Verification items for the finished model (mm, model axes). A direction names the side the tool comes from. Give positions to 0.01 mm unless a question says otherwise; leave off trailing zeros. Write each loop counter-clockwise with the first axis right and the second up, starting at its lowest first coordinate (ties: lowest second). Pieces come first, ordered by that corner, then holes. Notation, with made-up numbers: M 87,11.5 L 128,11.5 A12 cw 128,24.5 Z; hole C 16.5,52.25 d9. An arc over 180 degrees is marked long. Answer as a JSON object with one key per item and string values.
```python
from build123d import *

# Parameters (mm, degrees)
F0_W          = 76.2
F0_H          = 50.8
F1_DEPTH      = 50.8
F2_R          = 5.08
F3_R          = 6.35
F4_DEPTH      = 25.4
F4_DEPTH_BACK = 25.4
F5_SIZE       = 5.08


with BuildPart() as f1:
    # F0 (on Front) → F1 (new body)
    with BuildSketch(Plane.XZ):
        with Locations((38.1, 25.4)):
            Rectangle(F0_W, F0_H)
    extrude(amount=F1_DEPTH)

    # F2
    f2_edges = [f1.edges().sort_by_distance(p)[0] for p in [
        (0, -25.4, 50.8),
        (38.1, -50.8, 50.8),
        (0, -50.8, 25.4),
        (0, 0, 25.4),
    ]]
    fillet(f2_edges, radius=F2_R)

    # F3 (on face) → F4 (cut, two sides)
    with BuildSketch(Plane(origin=(0, 0, 0), x_dir=(0, -1, 0), z_dir=(-1, 0, 0))) as f4_sk:
        with Locations((30.48, 20.32)):
            Circle(F3_R)
    extrude(amount=-F4_DEPTH, mode=Mode.SUBTRACT)
    extrude(f4_sk.sketch, amount=-F4_DEPTH_BACK, mode=Mode.SUBTRACT)

    # F5
    f5_edges = [f1.edges().sort_by_distance(p)[0] for p in [
        (76.2, -50.8, 22.86),
        (76.2, -25.4, 0),
        (76.2, 0, 25.4),
    ]]
    chamfer(f5_edges, length=F5_SIZE)


solid = f1.part
```
1) Section check B-B on z = 20.32. Record the boundary of the cut face in (x, y), and give its area (3 significant figures).
Completed:
{"outline": "M 0,-45.72 A5.08 ccw 5.08,-50.8 L 71.12,-50.8 L 76.2,-45.72 L 76.2,-5.08 L 71.12,0 L 5.08,0 A5.08 ccw 0,-5.08 L 0,-24.13 L 25.4,-24.13 L 25.4,-36.83 L 0,-36.83 Z", "area": "3,510 mm2"}
2) Section check C-C on y = -4. Record the boundary of the cut face in (x, z).
Completed:
{"outline": "M 0.12,0 L 71.12,0 L 75.12,4 L 75.12,46.8 L 71.12,50.8 L 5.08,50.8 A5.08 ccw 0.12,46.8 Z"}
3) Release check for a two-part mould opening along Z. For faces 1 (the face through (0, -21, 23)), 2 (the face through (25.4, -30, 20)), 3 (the face through (1.449, -23.18, 49.272)) record: pulls with the +Z half, pulls with the -Z half, needs draft (parallel to the pull), parting line crosses it, or undercut.
Completed:
{"face 1": "needs draft", "face 2": "undercut", "face 3": "pulls with the +Z half"}
4) Thickness scan on L1, parallel to Z at x = 13.5, y = -30.48; L2, parallel to Y at x = 9, z = 20; L3, parallel to X at y = -4, z = 42. Record the ranges inside material, lowest first.
Completed:
{"L1": "z = 0 to 13.97, 26.67 to 50.8", "L2": "y = -50.8 to -36.82, -24.14 to 0", "L3": "x = 0.12 to 75.12"}
5) Section check A-A on y = -30.48. Record the boundary of the cut face in (x, z).
Completed:
{"outline": "M 0,0 L 71.12,0 L 76.2,5.08 L 76.2,45.72 L 71.12,50.8 L 5.08,50.8 A5.08 ccw 0,45.72 L 0,26.67 L 25.4,26.67 L 25.4,13.97 L 0,13.97 Z"}
6) Access from +Z, -Z, +X, -X, +Y, -Y to the whole of each face (thin tool, end or side, straight path). Record for faces 4 (the face through (38, -50.8, 23)), 5 (the face through (12.522, -24.136, 20.599)).
Completed:
{"face 4": "+Z, -Z, +X, -X, -Y", "face 5": "-X"}
7) Go/stop test with a flat-tipped pin: pin 1 (6.5 mm diameter, centred on y = -31.5, z = 19.5, fed in from -X). Record where the tip stops, or that it passes through.
Completed:
{"pin 1": "stops at x = 25.4"}
